Work out the finished part from the listing and answer in its coordinate system (mm). A direction names the side the tool comes from. Round coordinates to 2 decimals unless told otherwise and drop trailing zeros. Write each loop counter-clockwise with the first axis right and the second up, starting at its lowest first coordinate (ties: lowest second). Pieces come first, ordered by that corner, then holes. Notation, with made-up numbers: (-13, -8.5) - (46, -8.5) arc R26 cw to (46, 17.5) - close; hole circle Ø3 at (13.25, -20). An arc over 180 degrees is marked (long way). Answer as a JSON object with one key per item and string values.
Autodesk Inventor part; units mm, degrees
ref_plane "YZ Plane" through (0, 0, 0) normal (1, 0, 0) x (0, 1, 0)
ref_plane "XZ Plane" through (0, 0, 0) normal (0, 1, 0) x (-1, 0, 0)
ref_plane "XY Plane" through (0, 0, 0) normal (0, 0, 1) x (1, 0, 0)
sketch "Sketch1" plane through (0, 0, 0) normal (0, 1, 0) x (-1, 0, 0)
  line L0 (0, 0) -> (0, -100)
  line L1 (10, -100) -> (10, 0)
  circle A0 centre (5, -84.5) radius 2.6
  circle A1 centre (5, -15.5) radius 2.6
  circle A2 centre (5, -1) radius 3
  line L2 (10, 0) -> (10, 4)
  line L3 (10, 4) -> (0, 4)
  line L4 (0, 4) -> (0, 0)
  line L5 (10, -100) -> (10, -104)
  line L6 (10, -104) -> (0, -104)
  line L7 (0, -104) -> (0, -100)
  circle A3 centre (5, -99) radius 3
  circle A4 centre (5, -26) radius 2
  arc A5 (7, -34) -> (3, -34) centre (5, -34) ccw
  arc A6 (3, -42) -> (7, -42) centre (5, -42) ccw
  circle A7 centre (5, -50) radius 2
  arc A8 (7, -58) -> (3, -58) centre (5, -58) ccw
  arc A9 (3, -66) -> (7, -66) centre (5, -66) ccw
  circle A10 centre (5, -74) radius 2
  line L8 (7, -34) -> (7, -42)
  line L9 (3, -34) -> (3, -42)
  line L10 (7, -58) -> (7, -66)
  line L11 (3, -58) -> (3, -66)
  line L12 (5, -21) -> (10, -21)
  line L13 (5, -21) -> (0, -21)
  line L14 (5, -11.5) -> (10, -11.5)
  line L15 (5, -11.5) -> (0, -11.5)
  line L16 (5, -79) -> (10, -79)
  line L17 (5, -79) -> (0, -79)
  line L18 (5, -88.5) -> (10, -88.5)
  line L19 (5, -88.5) -> (0, -88.5)
  dimension "d0" = 100
  dimension "d1" = 10
  dimension "d4" = 5.2
  dimension "d7" = 5.2
  dimension "d9" = 6
  dimension "d10" = 4
  dimension "d11" = 4
  dimension "d13" = 6
  dimension "d20" = 4
  dimension "d21" = 4
  dimension "d22" = 4
  dimension "d23" = 4
  dimension "d24" = 4
  dimension "d25" = 4
  dimension "d26" = 4
  dimension "d27" = 5.5
  dimension "d28" = 4
  dimension "d29" = 5.5
  dimension "d30" = 4
extrude "Extrusion1" add sketch "Sketch1" along normal blind 3 contours L4 L3 L2 L1 L14 L15 L0 | L13 L12 L1 L16 L17 L0 | L19 L18 L1 L5 L6 L7 L0
extrude "Extrusion2" add sketch "Sketch1" along normal blind 6.2 contours L15 L14 L1 L12 L13 L0 | L17 L16 L1 L18 L19 L0 | A2 | A3
properties part number "roller_holder_2"
Item 1: Each of these flat-tipped pins is pushed along its axis until it touches: P1, Ø3, axis at y = 1, z = -71.5, coming from the +X side; P2, Ø3, axis at x = -5, z = -50, coming from the +Y side; P3, Ø5, axis at x = -4.5, z = -50.5, coming from the +Y side; P4, Ø1, axis at x = -7, y = 4, coming from the -Z side. Where does it stop, or does it pass through?
Results found:
{"P1": "x = 0", "P2": "through", "P3": "y = 3", "P4": "z = -101.6"}
Item 2: A cutting plane is placed at C-C (z = -1). Write down the section's boundary in (x, y), and give its area (3 significant figures).
Results found:
{"outline": "(-10, 0) - (0, 0) - (0, 3) - (-2, 3) - (-2, 6.2) - (-8, 6.2) - (-8, 3) - (-10, 3) - close", "area": "49.2 mm²"}
Item 3: Consider line 1 along Z through (x, y) = (-5, 4.5); line 2 along Z through (x, y) = (-6, 6); line 3 along Y through (x, z) = (-2.25, -37). Determine where each line is inside the solid, lowest interval first.
Results found:
{"line 1": "-102 to -96, -88.5 to -87.1, -81.9 to -79, -21 to -18.1, -12.9 to -11.5, -4 to 2", "line 2": "-101.83 to -96.17, -88.5 to -86.9, -82.1 to -79, -21 to -17.9, -13.1 to -11.5, -3.83 to 1.83", "line 3": "0 to 3"}
Item 4: A cutting plane is placed at B-B (x = -5). Give the number of separate pieces and of enclosed holes in the cut face, and give its area (3 significant figures).
Results found:
{"separate pieces": "8", "enclosed holes": "0", "area": "251 mm²"}
Item 5: For faces 1 (the cylindrical face through (-5, 1, -44)), 2 (the flat face through (-10, 2, -51)), 3 (the flat face through (-5, 6.2, -1)), 4 (the flat face through (-5, 3, -94)), 5 (the flat face through (-5, 5, -88.5)), determine the directions among +Z, -Z, +X, -X, +Y, -Y from which every point of the face is accessible in a straight line to the end or side of a thin tool.
Results found:
{"face 1": "+Y, -Y", "face 2": "+Z, -Z, -X, +Y, -Y", "face 3": "+Z, -Z, +X, -X, +Y", "face 4": "+Y", "face 5": "+X, -X, +Y"}
Item 6: A cutting plane is placed at D-D (x = -9). Write down the section's boundary in (y, z), and give its area (3 significant figures).
Results found:
{"outline": "(0, -104) - (3, -104) - (3, -88.5) - (6.2, -88.5) - (6.2, -79) - (3, -79) - (3, -21) - (6.2, -21) - (6.2, -11.5) - (3, -11.5) - (3, 4) - (0, 4) - close", "area": "385 mm²"}
Item 7: A cutting plane is placed at A-A (z = -84.5). Write down the section's boundary in (x, y), and give its area (3 significant figures).
Results found:
{"outline": "(-10, 0) - (-7.6, 0) - (-7.6, 6.2) - (-10, 6.2) - close; (-2.4, 0) - (0, 0) - (0, 6.2) - (-2.4, 6.2) - close", "area": "29.8 mm²"}
Item 8: Determine the mould class of faces 6 (the flat face through (-7, 1, -62)), 7 (the flat face through (-3, 1, -62)), 8 (the flat face through (-5, 5, -21)), 9 (the cylindrical face through (-4.35, 4.58, -96.07)) for opening direction X: pulls with the +X half, pulls with the -X half, needs draft (parallel to the pull), parting line crosses it, or undercut.
Results found:
{"face 6": "undercut", "face 7": "undercut", "face 8": "needs draft", "face 9": "parting line crosses it"}
